```python
from build123d import *

# Parameters (mm, degrees)
SKETCH1_W          = 44.45
SKETCH1_H          = 28.575
EXTRUDE1_DEPTH     = 38.1
SKETCH2_R          = 2.5527
SKETCH2_R_2        = 2.0193
CUT_EXTRUDE1_DEPTH = 66.145553379
SKETCH3_R          = 2.794
CUT_EXTRUDE2_DEPTH = 66.145553379
SKETCH4_W          = 8.128
SKETCH4_H          = 1.524
EXTRUDE2_DEPTH     = 14.732
SKETCH5_R          = 3.048
CUT_EXTRUDE3_DEPTH = 61.501738992


with BuildPart() as part:
    # Sketch1 → Extrude1 (new body)
    with BuildSketch(Plane(origin=(0, 0, 0), x_dir=(1, 0, 0), z_dir=(0, 1, 0))):
        with Locations((22.225, 14.2875)):
            Rectangle(SKETCH1_W, SKETCH1_H)
    extrude(amount=EXTRUDE1_DEPTH)

    # Sketch2 → Cut-Extrude1 (cut, through all)
    with BuildSketch(Plane(origin=(0, 38.1, 0), x_dir=(-1, 0, 0), z_dir=(0, 1, 0))):
        with Locations(Location((-22.225, -14.2875, 0), (0, 0, 90))):
            Circle(SKETCH2_R)
        with Locations(Location((-22.225, -24.511, 0), (0, 0, 90))):
            Circle(SKETCH2_R_2)
        with Locations(Location((-22.225, -4.064, 0), (0, 0, 90))):
            Circle(SKETCH2_R_2)
    extrude(amount=-CUT_EXTRUDE1_DEPTH, mode=Mode.SUBTRACT)

    # Sketch3 → Cut-Extrude2 (cut, through all)
    with BuildSketch(Plane(origin=(0, 0, -28.575), x_dir=(-1, 0, 0), z_dir=(0, 0, -1))):
        with Locations((-33.274, 15.748)):
            Circle(SKETCH3_R)
        with Locations((-11.176, 15.748)):
            Circle(SKETCH3_R)
    extrude(amount=-CUT_EXTRUDE2_DEPTH, mode=Mode.SUBTRACT)

    # Sketch4 → Extrude2 (add)
    with BuildSketch(Plane.XY):
        with Locations((11.684, 28.702)):
            Rectangle(SKETCH4_W, SKETCH4_H)
        with Locations((32.766, 28.702)):
            Rectangle(SKETCH4_W, SKETCH4_H)
    extrude(amount=EXTRUDE2_DEPTH)

    # Sketch5 → Cut-Extrude3 (cut, through all)
    with BuildSketch(Plane(origin=(0, 29.464, 0), x_dir=(-1, 0, 0), z_dir=(0, 1, 0))):
        with Locations(Location((-11.684, 9.271, 0), (0, 0, 90))):
            Circle(SKETCH5_R)
        with Locations(Location((-32.766, 9.271, 0), (0, 0, 90))):
            Circle(SKETCH5_R)
    extrude(amount=-CUT_EXTRUDE3_DEPTH, mode=Mode.SUBTRACT)


solid = part.part
```
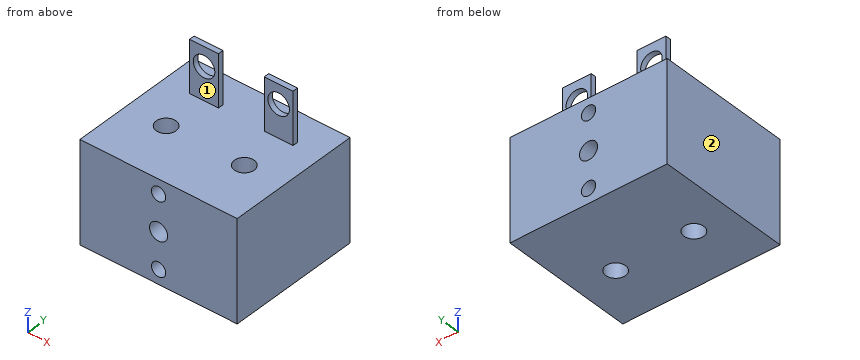
The model under review builds one solid part; all positions refer to its coordinate system, in mm. Face numbers are marked on the shaded views. A direction names the side the tool comes from. Round coordinates to 2 decimals unless told otherwise and drop trailing zeros. Write each loop counter-clockwise with the first axis right and the second up, starting at its lowest first coordinate (ties: lowest second). Pieces come first, ordered by that corner, then holes. Notation, with made-up numbers: M 75.5,61.5 L 133.5,61.5 A17 ccw 133.5,67.5 Z; hole C -32.75,68 d9. An arc over 180 degrees is marked long. Use CSV: the item, a comma, the result in double quotes. Start each with the question number.
(1) We need section D-D, the plane x = 21. State the section outline as (y, z) points (3 decimals), then the cut area to 3 significant figures.
(2) We need section A-A, the plane z = 2. State the section outline as (x, y) points.
(3) Clearance check with flat-ended pins moving along their axes: P1, Ø0.5, axis at y = 28.5, z = 6.5, coming from the +X side; P2, Ø4, axis at x = 34.5, z = 4.5, coming from the -Y side; P3, Ø3, axis at x = 29, y = 25, coming from the +Z side; P4, Ø3.5, axis at x = 32.766, z = 9.271, coming from the -Y side. State where each tip first meets the part, or that it passes through.
(4) We need section B-B, the plane x = 34. State the section outline as (y, z) points (3 decimals).
(5) For line 1 along X through (y, z) = (29, 9); line 2 along Z through (x, y) = (20.5, 21.5) (3 decimals); line 3 along X through (y, z) = (28, 4), list the stretches that pass through material, from the lowest coordinate up.
(6) We need section C-C, the plane z = -13.5. State the section outline as (x, y) points.
(7) Tool access review of the marked faces 1 and 2: name each direction out of +Z, -Z, +X, -X, +Y, -Y from which nothing blocks a thin tool from reaching the whole face with its end or side.
Findings:
1,outline,"M 0,-28.575 L 38.1,-28.575 L 38.1,-26.116 L 0,-26.116 Z; M 0,-22.906 L 38.1,-22.906 L 38.1,-16.527 L 0,-16.527 Z; M 0,-12.048 L 38.1,-12.048 L 38.1,-5.669 L 0,-5.669 Z; M 0,-2.459 L 38.1,-2.459 L 38.1,0 L 0,0 Z"
1,area,"673 mm^2"
2,outline,"M 7.62,27.94 L 15.75,27.94 L 15.75,29.46 L 7.62,29.46 Z; M 28.7,27.94 L 36.83,27.94 L 36.83,29.46 L 28.7,29.46 Z"
3,P1,"x = 36.83"
3,P2,"y = 27.94"
3,P3,"z = 0"
3,P4,"through"
4,outline,"M 0,-28.575 L 13.05,-28.575 L 13.05,0 L 0,0 Z; M 18.446,-28.575 L 38.1,-28.575 L 38.1,0 L 29.464,0 L 29.464,6.484 L 27.94,6.484 L 27.94,0 L 18.446,0 Z; M 27.94,12.058 L 29.464,12.058 L 29.464,14.732 L 27.94,14.732 Z"
5,line 1,"7.62 to 8.65, 14.72 to 15.75, 28.7 to 29.73, 35.8 to 36.83"
5,line 2,"-28.575 to -25.561, -23.461 to -16.169, -12.406 to -5.114, -3.014 to 0"
5,line 3,"7.62 to 15.75, 28.7 to 36.83"
6,outline,"M 0,0 L 19.8,0 L 19.8,38.1 L 0,38.1 Z; M 24.65,0 L 44.45,0 L 44.45,38.1 L 24.65,38.1 Z; hole C 11.18,15.75 d5.59; hole C 33.27,15.75 d5.59"
7,face 1,"+Z, +X, -X, -Y"
7,face 2,"+Z, -Z, -X, +Y, -Y"
